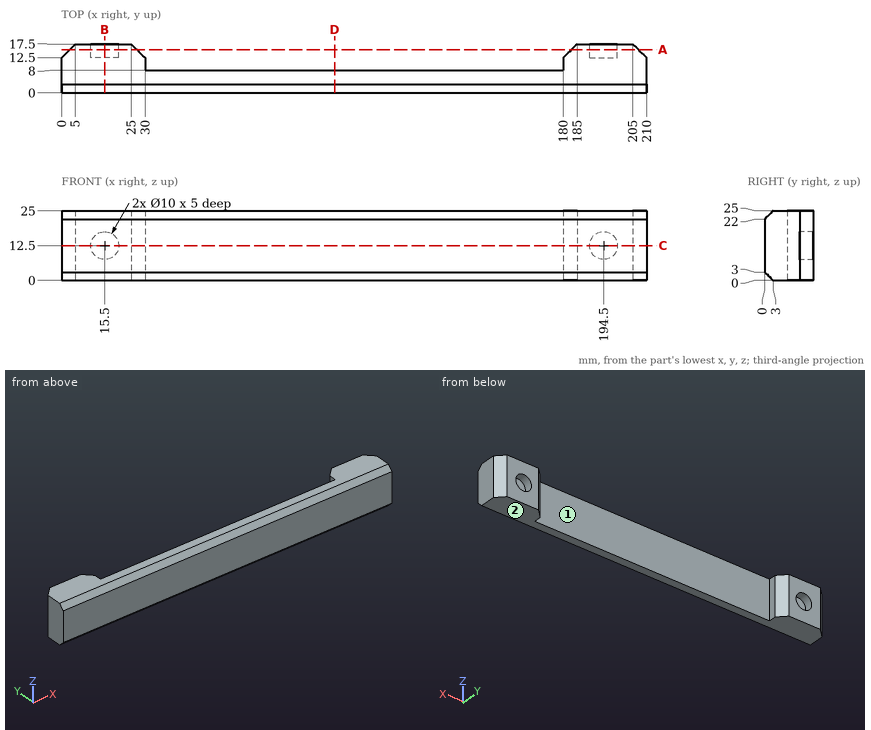
Study the drawing (mm; zero at the part's minimum x, y, z) and answer. Coordinates: 2 decimals unless noted, no trailing zeros. Loops run counter-clockwise (first coordinate to the right, second up) from the corner with the lowest first, then second, coordinate; pieces in that order, holes last. Notation, with made-up numbers: (61.25, -31) -> (116.25, -31) arc R18 ccw to (116.25, -27) -> close; hole circle Ø10 at (77.5, 84). An arc over 180 degrees is marked (long way). Answer in a Markdown table with one row per item. Add a question column.
1. Determine the mould class of the marked faces 1 and 2 for opening direction X: +X half, -X half, draft (parallel to the pull), parting line (faces both ways), or undercut.
2. Flat-ended cylindrical pins translate along their axes: P1, Ø3, axis at x = 193, z = 11, coming from the +Y side; P2, Ø1.5, axis at y = 6.5, z = 8, coming from the -X side; P3, Ø4, axis at x = 101, y = 10.5, coming from the +Z side. Find the tip coordinate at first contact, or state that the pin passes through.
3. The part is cut by section D-D, the plane x = 98. Write down the section's boundary in (y, z), then the cut area to 3 significant figures.
4. The part is cut by section A-A, the plane y = 15.5. Write down the section's boundary in (x, z).
5. The part is cut by section C-C, the plane z = 12.5. Write down the section's boundary in (x, y).
6. The part is cut by section B-B, the plane x = 15.5. Write down the section's boundary in (y, z).
7. Consider line 1 (X direction, y = 9.75, z = 14); line 2 (Z direction, x = 194.5, y = 15.85); line 3 (X direction, y = 14.6, z = 12.5). Determine where each line is inside the solid, lowest interval first. Write a range as [from, to].
Answer below:
| question | item | result |
|---|---|---|
| 1 | face 1 | undercut |
| 1 | face 2 | draft |
| 2 | P1 | y = 12.5 |
| 2 | P2 | x = 0 |
| 2 | P3 | through |
| 3 | outline | (0, 3) -> (3, 0) -> (8, 0) -> (8, 25) -> (3, 25) -> (0, 22) -> close |
| 3 | area | 191 mm2 |
| 4 | outline | (3, 0) -> (27, 0) -> (27, 25) -> (3, 25) -> close; (183, 0) -> (207, 0) -> (207, 25) -> (183, 25) -> close; hole circle Ø10 at (15.5, 12.5); hole circle Ø10 at (194.5, 12.5) |
| 5 | outline | (0, 0) -> (210, 0) -> (210, 12.5) -> (205, 17.5) -> (199.5, 17.5) -> (199.5, 12.5) -> (189.5, 12.5) -> (189.5, 17.5) -> (185, 17.5) -> (180, 12.5) -> (180, 8) -> (30, 8) -> (30, 12.5) -> (25, 17.5) -> (20.5, 17.5) -> (20.5, 12.5) -> (10.5, 12.5) -> (10.5, 17.5) -> (5, 17.5) -> (0, 12.5) -> close |
| 6 | outline | (0, 3) -> (3, 0) -> (17.5, 0) -> (17.5, 7.5) -> (12.5, 7.5) -> (12.5, 17.5) -> (17.5, 17.5) -> (17.5, 25) -> (3, 25) -> (0, 22) -> close |
| 7 | line 1 | [0, 30], [180, 210] |
| 7 | line 2 | [0, 7.5], [17.5, 25] |
| 7 | line 3 | [2.1, 10.5], [20.5, 27.9], [182.1, 189.5], [199.5, 207.9] |
